Check sheet for the modelled part. Datum: model origin and axes. Units: mm. Give positions to 0.01 mm unless a question says otherwise; leave off trailing zeros. Loops run counter-clockwise (first coordinate to the right, second up) from the corner with the lowest first, then second, coordinate; pieces in that order, holes last. Notation, with made-up numbers: M -8.5,-6.5 L 27.5,-6.5 A10 ccw 27.5,9.5 Z; hole C 37,-31.75 d2. An arc over 180 degrees is marked long. Use one line per item in the form item = value.
Autodesk Inventor part; units mm, degrees
ref_plane "YZ Plane" through (0, 0, 0) normal (1, 0, 0) x (0, 1, 0)
ref_plane "XZ Plane" through (0, 0, 0) normal (0, 1, 0) x (-1, 0, 0)
ref_plane "XY Plane" through (0, 0, 0) normal (0, 0, 1) x (1, 0, 0)
sketch "Sketch1" plane through (0, 0, 0) normal (0, 1, 0) x (-1, 0, 0)
  line L0 (18.5, 46.85) -> (-18.5, 46.85)
  line L1 (-18.5, 46.85) -> (-18.5, -46.85)
  line L2 (-18.5, -46.85) -> (18.5, -46.85)
  line L3 (18.5, -46.85) -> (18.5, 46.85)
  line L4 (18.5, 46.85) -> (-18.5, -46.85) construction
  line L5 (-18.5, 46.85) -> (18.5, -46.85) construction
  point P0 (0, 0)
  dimension "d0" = 93.7
  dimension "d1" = 37
extrude "Extrusion1" add sketch "Sketch1" along normal blind 12
sketch "Sketch2" plane through (18.5, 0, 46.85) normal (1, 0, 0) x (0, 0, -1)
  line L0 (5, 3.5) -> (18, 3.5)
  line L1 (18, 3.5) -> (18, 8.5)
  line L2 (18, 8.5) -> (5, 8.5)
  line L3 (5, 8.5) -> (5, 3.5)
  line L4 (5, 3.5) -> (18, 8.5) construction
  line L5 (18, 3.5) -> (5, 8.5) construction
  line L6 (23, 3.5) -> (36, 3.5)
  line L7 (36, 3.5) -> (36, 8.5)
  line L8 (36, 8.5) -> (23, 8.5)
  line L9 (23, 8.5) -> (23, 3.5)
  line L10 (23, 3.5) -> (36, 8.5) construction
  line L11 (36, 3.5) -> (23, 8.5) construction
  line L12 (41, 3.5) -> (54, 3.5)
  line L13 (54, 3.5) -> (54, 8.5)
  line L14 (54, 8.5) -> (41, 8.5)
  line L15 (41, 8.5) -> (41, 3.5)
  line L16 (41, 3.5) -> (54, 8.5) construction
  line L17 (54, 3.5) -> (41, 8.5) construction
  line L18 (59, 3.5) -> (72, 3.5)
  line L19 (72, 3.5) -> (72, 8.5)
  line L20 (72, 8.5) -> (59, 8.5)
  line L21 (59, 8.5) -> (59, 3.5)
  line L22 (59, 3.5) -> (72, 8.5) construction
  line L23 (72, 3.5) -> (59, 8.5) construction
  line L24 (0, 0) -> (0, 12)
  point P0 (46.85, 0)
  point P1 (11.5, 6)
  point P2 (29.5, 6)
  point P3 (47.5, 6)
  point P4 (65.5, 6)
  point P5 (0, 6)
  point P6 (54, 6)
  dimension "d4" = 5
  dimension "d5" = 5
  dimension "d6" = 5
  dimension "d7" = 5
  dimension "d8" = 13
  dimension "d9" = 5
extrude "Extrusion2" cut sketch "Sketch2" against normal blind 12
sketch "Sketch3" plane through (18.5, 0, -46.85) normal (0, 0, -1) x (-1, 0, 0)
  circle A0 centre (18.5, 6) radius 3.5
  point P0 (18.5, 0)
  dimension "d12" = 7
extrude "Extrusion3" add sketch "Sketch3" along normal blind 5
equation "\"d5\" = d4"
equation "\"d6\" = d5"
properties part number "USBextender"
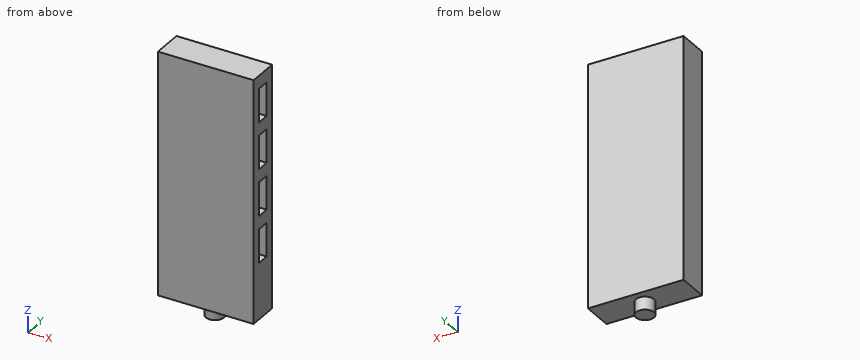
1) Section check C-C (x = 0). Record the cut outline in (y, z).
Evaluation:
outline = M 0,-46.85 L 2.5,-46.85 L 2.5,-51.85 L 9.5,-51.85 L 9.5,-46.85 L 12,-46.85 L 12,46.85 L 0,46.85 Z
2) Section check D-D (y = 1.5). Record the cut outline in (x, z).
Evaluation:
outline = M -18.5,-46.85 L 18.5,-46.85 L 18.5,46.85 L -18.5,46.85 Z
3) Section check A-A (z = 12.5). Record the cut outline in (x, y).
Evaluation:
outline = M -18.5,0 L 18.5,0 L 18.5,3.5 L 6.5,3.5 L 6.5,8.5 L 18.5,8.5 L 18.5,12 L -18.5,12 Z
4) Scan lines: line 1 (Z direction, x = 7, y = 6.25); line 2 (Y direction, x = 10, z = 16); line 3 (Z direction, x = -10, y = 4.75). Record each from-to range of solid material in increasing order.
Evaluation:
line_1 = -46.85 to -25.15, -12.15 to -7.15, 5.85 to 10.85, 23.85 to 28.85, 41.85 to 46.85
line_2 = 0 to 3.5, 8.5 to 12
line_3 = -46.85 to 46.85
5) Depth check by flat-ended pin: pin 1 Ø2 at (x, y) = (13.5, 7) entering from -Z; pin 2 Ø5.5 at (y, z) = (7, 33) entering from +X; pin 3 Ø1.5 at (y, z) = (6.5, -21) entering from +X. Enter the tip coordinate at first touch or a pass-through.
Evaluation:
pin_1 = -46.85
pin_2 = 18.5
pin_3 = 6.5
6) Section check B-B (y = 6). Record the cut outline in (x, z), then the cut area to 3 significant figures.
Evaluation:
outline = M -18.5,-46.85 L -3.5,-46.85 L -3.5,-51.85 L 3.5,-51.85 L 3.5,-46.85 L 18.5,-46.85 L 18.5,-25.15 L 6.5,-25.15 L 6.5,-12.15 L 18.5,-12.15 L 18.5,-7.15 L 6.5,-7.15 L 6.5,5.85 L 18.5,5.85 L 18.5,10.85 L 6.5,10.85 L 6.5,23.85 L 18.5,23.85 L 18.5,28.85 L 6.5,28.85 L 6.5,41.85 L 18.5,41.85 L 18.5,46.85 L -18.5,46.85 Z
area = 2,880 mm^2
